Input: part model. Units: mm. Frame: model coordinates. A direction names the side the tool comes from. Give positions to 0.01 mm unless a question says otherwise; leave off trailing zeros. Write each loop counter-clockwise with the first axis right and the second up, starting at its lowest first coordinate (ties: lowest second). Pieces come first, ordered by that corner, then holes.
```python
from build123d import *

# Parameters (mm, degrees)
SKETCH1_W           = 48
SKETCH1_H           = 15
SKETCH1_R           = 1.5
BOSS_EXTRUDE1_DEPTH = 2
SKETCH2_W           = 5
SKETCH2_H           = 5
BOSS_EXTRUDE2_DEPTH = 1


with BuildPart() as part:
    # Sketch1 → Boss-Extrude1 (new body)
    with BuildSketch(Plane.XY):
        with Locations((24, 7.5)):
            Rectangle(SKETCH1_W, SKETCH1_H)
        with Locations((6, 7.5)):
            Circle(SKETCH1_R, mode=Mode.SUBTRACT)
        with Locations(Location((42, 7.5, 0), (0, 0, 180))):
            Circle(SKETCH1_R, mode=Mode.SUBTRACT)
    extrude(amount=BOSS_EXTRUDE1_DEPTH)

    # Sketch2 → Boss-Extrude2 (add)
    with BuildSketch(Plane.XY.offset(2)):
        with Locations((24, 7.5)):
            Rectangle(SKETCH2_W, SKETCH2_H)
    extrude(amount=BOSS_EXTRUDE2_DEPTH)


solid = part.part
```
Q1. Section D-D, the plane x = 42.5. Return the cut outline in (y, z), then the cut area to 3 significant figures.
Q2. Mould query, pull axis Z, two halves, no side actions, for faces 6 (the flat face through (24, 8, 3)), 7 (the flat face through (24, 8, 0)), 8 (the flat face through (24, 5, 2.5)). Classes: +Z half, -Z half, draft (parallel to the pull), parting line (faces both ways), or undercut.
Q3. Access query for faces 1 (the flat face through (24, 10, 2.5)), 2 (the flat face through (26.5, 7.5, 2.5)), 3 (the flat face through (0, 7, 1)), 4 (the flat face through (21.5, 7.5, 2.5)), 5 (the flat face through (24, 0, 1)). Directions: +Z, -Z, +X, -X, +Y, -Y. A direction counts if a zero-diameter tool reaches every point of the face in a straight line with its end or side. Return the directions, or none.
Q4. Section A-A, the plane x = 6. Return the cut outline in (y, z).
Q5. Pin query (flat end, axial travel): pin 1 (0.8 mm diameter, centred on x = 23.5, z = 2.5, fed in from +Y); pin 2 (3 mm diameter, centred on x = 38, y = 8.5, fed in from +Z). Return the tip coordinate at first contact, or that it passes through.
Q6. Material intervals for line 1 along Y through (x, z) = (6, 1.2); line 2 along X through (y, z) = (8.5, 1.4); line 3 along X through (y, z) = (8.25, 2.4), sorted ascending.
Q7. Section B-B, the plane y = 7.5. Return the cut outline in (x, z), then the cut area to 3 significant figures.
Q8. Section C-C, the plane z = 0.45. Return the cut outline in (x, y).
Solutions:
1. outline: (0, 0) - (6.09, 0) - (6.09, 2) - (0, 2) - close; (8.91, 0) - (15, 0) - (15, 2) - (8.91, 2) - close
1. area: 24.3 mm2
2. face 6: +Z half
2. face 7: -Z half
2. face 8: draft
3. face 1: +Z, +X, -X, +Y
3. face 2: +Z, +X, +Y, -Y
3. face 3: +Z, -Z, -X, +Y, -Y
3. face 4: +Z, -X, +Y, -Y
3. face 5: +Z, -Z, +X, -X, -Y
4. outline: (0, 0) - (6, 0) - (6, 2) - (0, 2) - close; (9, 0) - (15, 0) - (15, 2) - (9, 2) - close
5. pin 1: stops at y = 10
5. pin 2: stops at z = 2
6. line 1: y = 0 to 6, 9 to 15
6. line 2: x = 0 to 4.88, 7.12 to 40.88, 43.12 to 48
6. line 3: x = 21.5 to 26.5
7. outline: (0, 0) - (4.5, 0) - (4.5, 2) - (0, 2) - close; (7.5, 0) - (40.5, 0) - (40.5, 2) - (26.5, 2) - (26.5, 3) - (21.5, 3) - (21.5, 2) - (7.5, 2) - close; (43.5, 0) - (48, 0) - (48, 2) - (43.5, 2) - close
7. area: 89.0 mm2
8. outline: (0, 0) - (48, 0) - (48, 15) - (0, 15) - close; hole circle Ø3 at (6, 7.5); hole circle Ø3 at (42, 7.5)
